Source: CAD feature listing. Evaluate the final solid. Frame: model axes, mm. A direction names the side the tool comes from. Coordinates: 2 decimals unless noted, no trailing zeros. Order: outer loops, then holes, each group sorted by start corner. A loop starts at its lowest first (then second) coordinate and runs counter-clockwise, first axis right, second up.
```python
from build123d import *

# Parameters (mm, degrees)
F0_R     = 285.75
F1_DEPTH = 762
F2_T     = -12.7
F3_R     = 36.5125
F4_DEPTH = 327.66
F5_R     = 36.5125
F6_DEPTH = 345.44


with BuildPart() as f1:
    # F0 (on Top) → F1 (new body)
    with BuildSketch(Plane.XY):
        Circle(F0_R)
    extrude(amount=F1_DEPTH)

    # F2
    f2_openings = [f1.faces().sort_by_distance(p)[0] for p in [
        (0, 0, 762),
    ]]
    offset(amount=F2_T, openings=f2_openings)

    # F3 (on Front) → F4 (cut)
    with BuildSketch(Plane.XZ):
        with Locations((0, 50.8)):
            Circle(F3_R)
    extrude(amount=F4_DEPTH, mode=Mode.SUBTRACT)

    # F5 (on Front) → F6 (cut)
    with BuildSketch(Plane.XZ):
        with Locations((0, 50.8)):
            Circle(F5_R)
    extrude(amount=-F6_DEPTH, mode=Mode.SUBTRACT)


solid = f1.part
```
Q1. Section query C-C on y = 20. Output: boundary loops of the cut face in (x, z), plus the area to 3 significant figures.
Solutions:
outline: (-285.05, 0) - (285.05, 0) - (285.05, 762) - (272.32, 762) - (272.32, 12.7) - (-272.32, 12.7) - (-272.32, 762) - (-285.05, 762) - close
area: 26,300 mm2
Q2. Section query B-B on z = 62. Output: boundary loops of the cut face in (x, y).
Solutions:
outline: (-34.75, -283.63) - (-34.75, -270.83) arc R273.05 cw to (-34.75, 270.83) - (-34.75, 283.63) arc R285.75 ccw to start; (34.75, -283.63) arc R285.75 ccw to (34.75, 283.63) - (34.75, 270.83) arc R273.05 cw to (34.75, -270.83) - close
Q3. Section query A-A on x = 0. Output: boundary loops of the cut face in (y, z).
Solutions:
outline: (-285.75, 0) - (285.75, 0) - (285.75, 14.29) - (273.05, 14.29) - (273.05, 12.7) - (-273.05, 12.7) - (-273.05, 14.29) - (-285.75, 14.29) - close; (-285.75, 87.31) - (-273.05, 87.31) - (-273.05, 762) - (-285.75, 762) - close; (273.05, 87.31) - (285.75, 87.31) - (285.75, 762) - (273.05, 762) - close
Q4. Pin query (flat end, axial travel): P1, Ø1.5, axis at y = 228.5, z = 331.5, coming from the -X side; P2, Ø1, axis at y = -29.5, z = 312.5, coming from the -X side; P3, Ø2, axis at y = -218.5, z = 142.5, coming from the +X side. Return the tip coordinate at first contact, or that it passes through.
Solutions:
P1: stops at x = -172.58
P2: stops at x = -284.27
P3: stops at x = 185.33
Q5. Pull-direction query (Y, two-part tool) for faces 3 (the cylindrical face through (-59.192, -266.557, 382.105)), 4 (the flat face through (147, -231, 762)), 5 (the cylindrical face through (-285.474, 12.564, 375.666)); classes: pulls with the +Y half, pulls with the -Y half, needs draft (parallel to the pull), parting line crosses it, or undercut.
Solutions:
face 3: undercut
face 4: needs draft
face 5: parting line crosses it
Q6. Material intervals for line 1 along Y through (x, z) = (0, 593); line 2 along Z through (x, y) = (0, 275.5); line 3 along Y through (x, z) = (-197.5, 244.5), sorted ascending.
Solutions:
line 1: y = -285.75 to -273.05, 273.05 to 285.75
line 2: z = 0 to 14.29, 87.31 to 762
line 3: y = -206.51 to -188.55, 188.55 to 206.51
Q7. Section query D-D on x = 162.5. Output: boundary loops of the cut face in (y, z).
Solutions:
outline: (-235.05, 0) - (235.05, 0) - (235.05, 762) - (219.43, 762) - (219.43, 12.7) - (-219.43, 12.7) - (-219.43, 762) - (-235.05, 762) - close
Q8. Set-up query: faces 1 (the cylindrical face through (34.826, -278.07, 61.767)), 2 (the flat face through (-4, 4, 12.7)). Return all of +Z, -Z, +X, -X, +Y, -Y with unobstructed straight access to the full face (end or side cutting, diameter ignored); none if empty.
Solutions:
face 1: +Y, -Y
face 2: +Z
